Design review of the part shown in the three views and the two pictorial views. Dimensions are in mm from the part's minimum x, y and z. A direction names the side the tool comes from. Give positions to 0.01 mm unless a question says otherwise; leave off trailing zeros. Loops run counter-clockwise (first coordinate to the right, second up) from the corner with the lowest first, then second, coordinate; pieces in that order, holes last.
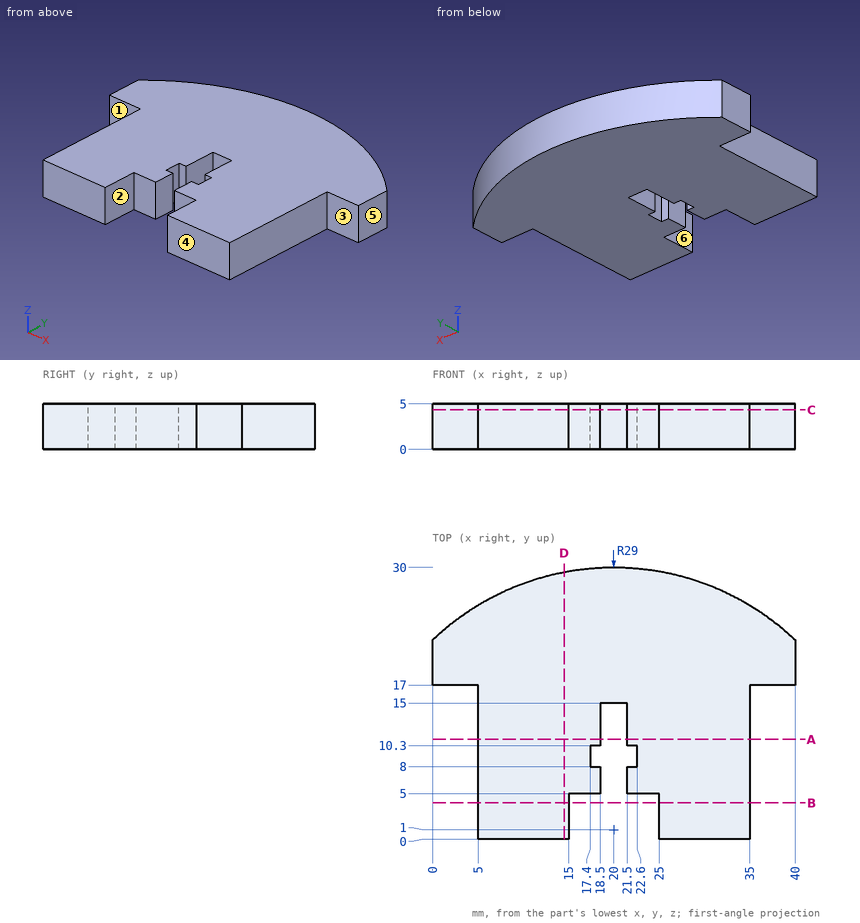
Q1. Tool access review of the marked faces 1, 2 and 3: name each direction out of +Z, -Z, +X, -X, +Y, -Y from which nothing blocks a thin tool from reaching the whole face with its end or side.
Results:
face 1: +Z, -Z, -X, -Y
face 2: +Z, -Z, -Y
face 3: +Z, -Z, +X, -Y
Q2. Take a section at B-B (y = 4). Give the boundary of the cut face in (x, z).
Results:
outline: (5, 0) - (15, 0) - (15, 5) - (5, 5) - close; (25, 0) - (35, 0) - (35, 5) - (25, 5) - close
Q3. Wall thickness on line 1 (X direction, y = 1.5, z = 4); line 2 (X direction, y = 12, z = 3.4); line 3 (Y direction, x = 20.5, z = 2.45): over which ranges is each line inside the solid? List them lowest first.
Results:
line 1: x = 5 to 15, 25 to 35
line 2: x = 5 to 18.5, 21.5 to 35
line 3: y = 15 to 30
Q4. Take a section at A-A (y = 11). Give the boundary of the cut face in (x, z), plus the area to 3 significant figures.
Results:
outline: (5, 0) - (18.5, 0) - (18.5, 5) - (5, 5) - close; (21.5, 0) - (35, 0) - (35, 5) - (21.5, 5) - close
area: 135 mm2
Q5. Insertion check: pin 1 (0.9 mm diameter, centred on x = 18, z = 3.5, fed in from +Y); pin 2 (0.6 mm diameter, centred on x = 18, z = 1.5, fed in from -Y); pin 3 (1.5 mm diameter, centred on y = 2.5, z = 2.5, fed in from +X). Each pin has a flat end and moves straight along its axis. Give the tip position at first contact, or say it passes through.
Results:
pin 1: stops at y = 29.96
pin 2: stops at y = 5
pin 3: stops at x = 35
Q6. Take a section at C-C (z = 4.35). Give the boundary of the cut face in (x, y).
Results:
outline: (0, 17) - (5, 17) - (5, 0) - (15, 0) - (15, 5) - (18.5, 5) - (18.5, 8) - (17.4, 8) - (17.4, 10.3) - (18.5, 10.3) - (18.5, 15) - (21.5, 15) - (21.5, 10.3) - (22.6, 10.3) - (22.6, 8) - (21.5, 8) - (21.5, 5) - (25, 5) - (25, 0) - (35, 0) - (35, 17) - (40, 17) - (40, 22) arc R29 ccw to (0, 22) - close
Q7. Draft analysis for pull direction X (two halves, no side actions). For the marked faces 4, 5 and 6, state which applies: pulls with the +X half, pulls with the -X half, needs draft (parallel to the pull), parting line crosses it, or undercut.
Results:
face 4: needs draft
face 5: pulls with the +X half
face 6: undercut
Q8. Take a section at D-D (x = 14.5). Give the boundary of the cut face in (y, z).
Results:
outline: (0, 0) - (29.47, 0) - (29.47, 5) - (0, 5) - close
